from build123d import *

# Parameters (mm, degrees)
CUT_EXTRUDE_1_DEPTH      = 132.165925626
CUT_EXTRUDE_1_DEPTH_BACK = 132.165925626
PATTERN_CIRCULAR_1_COUNT = 2
CUT_EXTRUDE_2_DEPTH      = 132.165925626


with BuildPart() as part:
    # Эскиз1 → Повернуть1 (revolve)
    with BuildSketch(Plane.XY, mode=Mode.PRIVATE) as revolve_1_sk:
        Polygon((0, 0), (-73.5, 0), (-73.5, 29), (-29, 55), (0, 55), align=None)
    revolve(revolve_1_sk.sketch.rotate(Axis((0, 0, 0), (0, -1, 0)), 270), axis=Axis((0, 0, 0), (0, -1, 0)))

    # Эскиз2 for По сечениям2 → По сечениям2 section 0
    with BuildSketch(Plane(origin=(0, 29, 0), x_dir=(-1, 0, 0), z_dir=(0, -1, 0))):
        with BuildLine():
            # circular arc as an exact rational Bezier (weights 1, cos(half-angle), 1)
            Bezier((39.466469787, -49.694809123), (86.422497659, 1.641217724), (45.380271287, 57.817652822), weights=[1, 0.773839067, 1])
            Bezier((45.380271287, 57.817652822), (34.990210983, 65.972666599), (22.410934831, 70), weights=[1, 0.984234087, 1])
            Bezier((22.410934831, 70), (39.972131567, 31.613018677), (20, -5.576629433), weights=[1, 0.895632627, 1])
            Bezier((20, -5.576629433), (14.31567319, -14.44600737), (5, -19.364916731), weights=[1, 0.96702533, 1])
            Bezier((5, -19.364916731), (11.820283108, -36.758324694), (25, -50), weights=[1, 0.979126148, 1])
            Bezier((25, -50), (32.393156545, -57.42791209), (39.466469787, -49.694809123), weights=[1, 0.690340696, 1])
        make_face()
    # Эскиз3 for По сечениям2 → По сечениям2 section 1
    with BuildSketch(Plane(origin=(0, 80, 0), x_dir=(1, 0, 0), z_dir=(0, 1, 0))):
        with BuildLine():
            Bezier((-32.410934831, 65.968032435), (-39.322570908, 62.57225757), (-45.380271287, 57.817652822), weights=[1, 0.994556139, 1])
            Bezier((-45.380271287, 57.817652822), (-86.422497659, 1.641217724), (-39.466469787, -49.694809123), weights=[1, 0.773839067, 1])
            Bezier((-39.466469787, -49.694809123), (-30.797796987, -53.302893985), (-25.13120111, -45.815981695), weights=[1, 0.790811163, 1])
            Bezier((-25.13120111, -45.815981695), (-19.944058149, -40.248445108), (-15.802261293, -33.864916731), weights=[1, 0.99619641, 1])
            Bezier((-15.802261293, -33.864916731), (-27.58094632, -26.902479263), (-35, -15.405932001), weights=[1, 0.973224743, 1])
            Bezier((-35, -15.405932001), (-55.902003331, 25.987274602), (-32.410934831, 65.968032435), weights=[1, 0.877862587, 1])
        make_face()
    loft_2 = loft()

    # Эскиз6 → Вырез-Вытянуть1 (cut, two sides: drawn at the far end of the back side and taken through both)
    with BuildSketch(Plane(origin=(0, 0, 0), x_dir=(0, 0, -1), z_dir=(1, 0, 0)).offset(-CUT_EXTRUDE_1_DEPTH_BACK)):
        Polygon((67.391079811, 62), (-50.626182403, 80), (-50.626182403, 96.194321308), (67.391079811, 98.711918652), align=None)
    extrude(amount=CUT_EXTRUDE_1_DEPTH + CUT_EXTRUDE_1_DEPTH_BACK, mode=Mode.SUBTRACT)

    # Круговой массив1: По сечениям2 ×2 about axis
    pattern_circular_1_axis = Axis((0, 0, 0), (0, 1, 0))
    for i in range(1, PATTERN_CIRCULAR_1_COUNT):
        add(loft_2.rotate(pattern_circular_1_axis, i * 360 / PATTERN_CIRCULAR_1_COUNT))

    # Эскиз7 → Вырез-Вытянуть2 (cut, through all)
    with BuildSketch(Plane(origin=(0, 0, 0), x_dir=(0, 0, -1), z_dir=(1, 0, 0))):
        Polygon((50.626182403, 80), (50.626182403, 117.416831393), (-67.391079811, 118.791932979), (-67.391079811, 62), align=None)
    extrude(amount=CUT_EXTRUDE_2_DEPTH, mode=Mode.SUBTRACT)


solid = part.part
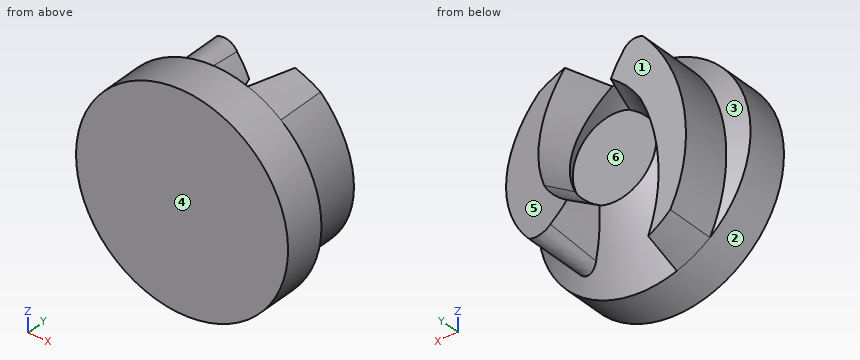
Design review of the part built by this model. Coordinates are the model's own, in mm. Face numbers are marked on the shaded views. A direction names the side the tool comes from. Coordinates: 2 decimals unless noted, no trailing zeros. Order: outer loops, then holes, each group sorted by start corner. A loop starts at its lowest first (then second) coordinate and runs counter-clockwise, first axis right, second up. Notation, with made-up numbers: (47, 25.25) -> (87, 25.25) arc R20 cw to (87, 38.25) -> close; hole circle Ø4 at (55, 39). An arc over 180 degrees is marked (long way). Use one line per item in the form item = value. Start each with the question number.
(1) The part is to be moulded in two halves that separate along X. For the marked faces 1, 2 and 3, say which applies: +X half, -X half, draft (parallel to the pull), parting line (faces both ways), or undercut.
(2) Insertion check: pin 1 (10 mm diameter, centred on x = 49.5, y = 47.5, fed in from -Z); pin 2 (4 mm diameter, centred on x = -37, z = 58, fed in from +Y); pin 3 (1 mm diameter, centred on y = 39.5, z = 14.5, fed in from -X). Each pin has a flat end and moves straight along its axis. Give the tip position at first contact, or say it passes through.
(3) For probe 1 along Y at (x, z) = (-5.5, -3.5); probe 2 along X at (y, z) = (67, 17.5); probe 3 along Y at (x, z) = (53.5, -22.5), list the stretches that pass through material, from the lowest coordinate up.
(4) Add section A-A on y = 18.5. State the section outline as (x, z) points.
(5) Add section B-B on x = 0. State the section outline as (y, z) points.
(6) For the marked faces 4, 5 and 6, list the 3-axis set-ups (+Z, -Z, +X, -X, +Y, -Y) from which the entire face can be reached by the end or side of a thin tool; tool diameter is ignored.
Answer block:
q1.face_1 = draft
q1.face_2 = parting line
q1.face_3 = undercut
q2.pin_1 = -43.65
q2.pin_2 = 32.92
q2.pin_3 = -58.94
q3.probe_1 = 0 to 55
q3.probe_2 = -57.93 to -27.85, 40.11 to 61.18
q3.probe_3 = 0 to 75.71
q4.outline = circle Ø147 at (0, 0)
q5.outline = (0, -73.5) -> (29, -73.5) -> (55, -29) -> (55, 29) -> (29, 73.5) -> (0, 73.5) -> close
q6.face_4 = +Z, -Z, +X, -X, -Y
q6.face_5 = +Z, +X, +Y
q6.face_6 = +Y
